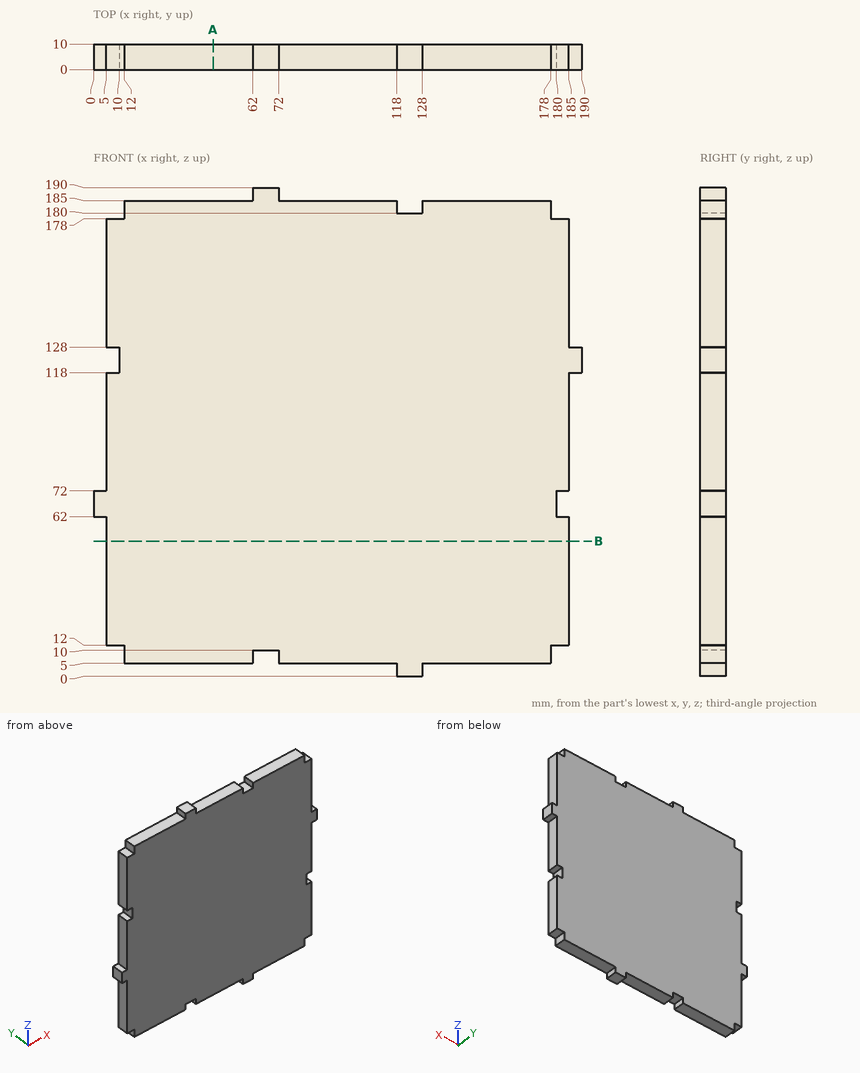
Could you check a few things on this drawing? It's one solid part, dimensions in mm from its lowest x, y, z. Give positions to 0.01 mm unless a question says otherwise; leave off trailing zeros. Write each loop counter-clockwise with the first axis right and the second up, starting at its lowest first coordinate (ties: lowest second). Pieces come first, ordered by that corner, then holes.
(1) Will these pins go through, and if not, where does the flat tip stop? pin 1 (5.5 mm diameter, centred on y = 4, z = 187, fed in from +X); pin 2 (3 mm diameter, centred on y = 7, z = 66, fed in from +X); pin 3 (6 mm diameter, centred on y = 3, z = 148.5, fed in from -X).
Output values:
pin 1: stops at x = 178
pin 2: stops at x = 180
pin 3: stops at x = 5
(2) If I drill on L1, parallel to Z at x = 160.5, y = 8.75; L2, parallel to Z at x = 124.5, y = 8.75, over which ranges is the centre line in solid material (lowest first)?
Output values:
L1: z = 5 to 185
L2: z = 0 to 180
(3) Imagine slicing it at B-B, the plane z = 52.5. Write out the boundary of the cut face in (x, y).
Output values:
outline: (5, 0) - (185, 0) - (185, 10) - (5, 10) - close
(4) Imagine slicing it at A-A, the plane x = 46.5. Write out the boundary of the cut face in (y, z).
Output values:
outline: (0, 5) - (10, 5) - (10, 185) - (0, 185) - close
